Solid Edge part; units mm, degrees
sketch "Sketch1" plane through (0, 0, 0) normal (0, 0, 1) x (1, 0, 0)
  circle A0 centre (0, 0) radius 10
extrude "Protrusion1" add sketch "Sketch1" along normal blind 3
sketch "Sketch2" plane through (0, 0, 0) normal (0, 0, -1) x (1, 0, 0)
  circle A0 centre (0, 0) radius 6.5
extrude "Protrusion2" add sketch "Sketch2" along normal blind 7.5
sketch "Sketch3" plane through (0, 0, -7.5) normal (0, 0, -1) x (1, 0, 0)
  line L0 (-3.5, 3.5707) -> (-3.5, -3.5707)
  arc A0 (-3.5, 3.5707) -> (-3.5, -3.5707) centre (0, 0) cw
extrude "Protrusion3" add sketch "Sketch3" along normal blind 8
sketch "Sketch4" plane through (0, 0, 3) normal (0, 0, 1) x (1, 0, 0)
  line L0 (-6.1644, 8.5) -> (6.1644, 8.5)
  arc A0 (6.1644, 8.5) -> (6.1644, -8.5) centre (0, 0) cw
  line L1 (-6.1644, -8.5) -> (6.1644, -8.5)
  arc A1 (-6.1644, -8.5) -> (-6.1644, 8.5) centre (0, 0) cw
extrude "Protrusion4" add sketch "Sketch4" along normal blind 5
sketch "Sketch5" plane through (0, 0, 8) normal (0, 0, 1) x (1, 0, 0)
  circle A0 centre (0, 0) radius 7.75
extrude "Protrusion5" add sketch "Sketch5" along normal blind 5
sketch "Sketch6" plane through (0, 0, 13) normal (0, 0, 1) x (1, 0, 0)
  circle A0 centre (0, 0) radius 5
extrude "Protrusion6" add sketch "Sketch6" along normal blind 12
chamfer "Chamfer1" distance 0.5 angle 45 1 edges at (-5, 0, 25)
properties part number "SHAFT2" material "4140 Steel"
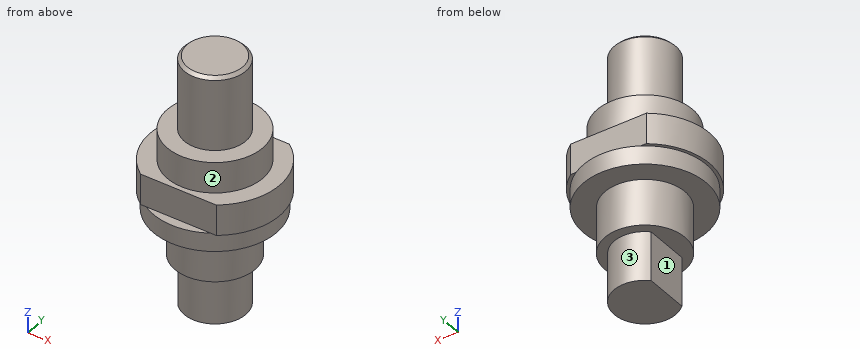
Work out the finished part from the listing and answer in its coordinate system (mm). Face numbers are marked on the shaded views. A direction names the side the tool comes from. Round coordinates to 2 decimals unless told otherwise and drop trailing zeros. Write each loop counter-clockwise with the first axis right and the second up, starting at its lowest first coordinate (ties: lowest second). Pieces come first, ordered by that corner, then holes. Notation, with made-up numbers: (19.5, 70.25) -> (69.5, 70.25) arc R27 cw to (69.5, 100.25) -> close; hole circle Ø11 at (80.25, 82.5). An arc over 180 degrees is marked (long way). Write each question's results on one line, items separated by ' | '.
Item 1: A cutting plane is placed at D-D, the plane x = 9. Determine the outline of the cut face in (y, z), plus the area to 3 significant figures.
Result set:
outline: (-5.41, 3) -> (-4.36, 3) -> (-4.36, 0) -> (4.36, 0) -> (4.36, 3) -> (5.41, 3) -> (5.41, 8) -> (-5.41, 8) -> close | area: 80.2 mm^2
Item 2: Which of the six approach directions +Z, -Z, +X, -X, +Y, -Y give full straight-line access (tool end or side, diameter ignored) to the marked faces 1, 2 and 3?
Result set:
face 1: -Z, -X, +Y, -Y | face 2: +Z | face 3: -Z
Item 3: A cutting plane is placed at B-B, the plane y = 0. Determine the outline of the cut face in (x, z), plus the area to 3 significant figures.
Result set:
outline: (-10.5, 3) -> (-10, 3) -> (-10, 0) -> (-6.5, 0) -> (-6.5, -7.5) -> (-3.5, -7.5) -> (-3.5, -15.5) -> (5, -15.5) -> (5, -7.5) -> (6.5, -7.5) -> (6.5, 0) -> (10, 0) -> (10, 3) -> (10.5, 3) -> (10.5, 8) -> (7.75, 8) -> (7.75, 13) -> (5, 13) -> (5, 24.5) -> (4.5, 25) -> (-4.5, 25) -> (-5, 24.5) -> (-5, 13) -> (-7.75, 13) -> (-7.75, 8) -> (-10.5, 8) -> close | area: 528 mm^2
Item 4: A cutting plane is placed at C-C, the plane z = 11. Determine the outline of the cut face in (x, y), plus the area to 3 significant figures.
Result set:
outline: circle Ø15.5 at (0, 0) | area: 189 mm^2
Item 5: A cutting plane is placed at A-A, the plane x = 0. Determine the outline of the cut face in (y, z), plus the area to 3 significant figures.
Result set:
outline: (-10, 0) -> (-6.5, 0) -> (-6.5, -7.5) -> (-5, -7.5) -> (-5, -15.5) -> (5, -15.5) -> (5, -7.5) -> (6.5, -7.5) -> (6.5, 0) -> (10, 0) -> (10, 3) -> (8.5, 3) -> (8.5, 8) -> (7.75, 8) -> (7.75, 13) -> (5, 13) -> (5, 24.5) -> (4.5, 25) -> (-4.5, 25) -> (-5, 24.5) -> (-5, 13) -> (-7.75, 13) -> (-7.75, 8) -> (-8.5, 8) -> (-8.5, 3) -> (-10, 3) -> close | area: 520 mm^2
Item 6: Find the intervals of material crossed by line 1 along Z through (x, y) = (6.25, -0.5); line 2 along X through (y, z) = (0.25, 23); line 3 along Z through (x, y) = (-7.5, -6.25), in increasing order. Write a range as [from, to].
Result set:
line 1: [-7.5, 13] | line 2: [-4.99, 4.99] | line 3: [0, 8]
Item 7: Flat-ended cylindrical pins translate along their axes: P1, Ø1.6, axis at x = -2, y = 9, coming from the +Z side; P2, Ø4, axis at x = 2, z = 6, coming from the -Y side; P3, Ø5, axis at x = 1.5, z = -7, coming from the -Y side. Find the tip coordinate at first contact, or state that the pin passes through.
Result set:
P1: z = 8 | P2: y = -8.5 | P3: y = -6.5
